Model file for the job. Use its own axes, mm. Give positions to 0.01 mm unless a question says otherwise; leave off trailing zeros. Order: outer loops, then holes, each group sorted by start corner. A loop starts at its lowest first (then second) coordinate and runs counter-clockwise, first axis right, second up. Notation, with made-up numbers: (65.5, 25) - (86.5, 25) arc R23 ccw to (86.5, 43) - close; hole circle Ø9 at (77, 18.25). An arc over 180 degrees is marked (long way). Return JSON: item names as keys, results as strings. Group by question number.
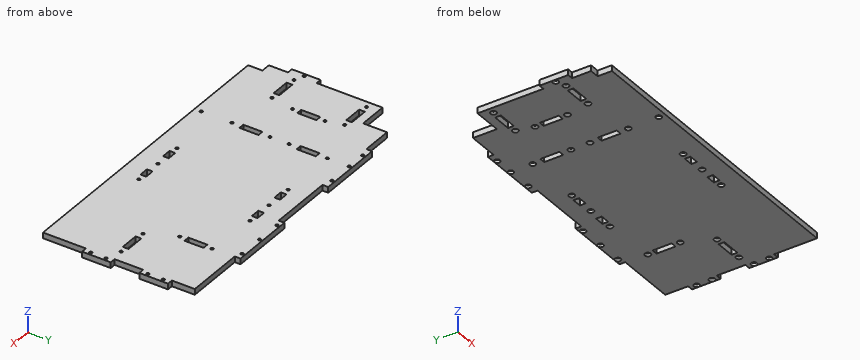
from build123d import *

# Parameters (mm, degrees)
ESQUISSE1_W             = 340
ESQUISSE1_H             = 165
BOSS_EXTRU_1_DEPTH      = 6
ESQUISSE2_W             = 6
ESQUISSE2_H             = 20
ESQUISSE2_W_2           = 68
ESQUISSE2_H_2           = 6
ESQUISSE2_H_3           = 45
ESQUISSE2_H_4           = 35
ESQUISSE2_H_5           = 30
ESQUISSE2_W_3           = 20
ENL_V_MAT_EXTRU_1_DEPTH = 6
ESQUISSE3_W             = 6
ESQUISSE3_H             = 20
ESQUISSE3_W_2           = 20
ESQUISSE3_H_2           = 6
ESQUISSE3_W_3           = 30
ESQUISSE3_H_3           = 25
ENL_V_MAT_EXTRU_2_DEPTH = 10
ESQUISSE5_R             = 1.5
ESQUISSE5_W             = 10
ESQUISSE5_H             = 6
ENL_V_MAT_EXTRU_4_DEPTH = 6
ESQUISSE7_R             = 1.5
ESQUISSE7_R_2           = 1.505
ESQUISSE7_W             = 10
ESQUISSE7_H             = 15
ENL_V_MAT_EXTRU_7_DEPTH = 378.969575495
ESQUISSE8_R             = 2.995
ESQUISSE8_R_2           = 3
ENL_V_MAT_EXTRU_9_DEPTH = 3


with BuildPart() as part:
    # Esquisse1 → Boss.-Extru.1 (new body)
    with BuildSketch(Plane.XY):
        with Locations((-170, 82.5)):
            Rectangle(ESQUISSE1_W, ESQUISSE1_H)
    extrude(amount=BOSS_EXTRU_1_DEPTH)

    # Esquisse2 → Enlèv. mat.-Extru.1 (cut)
    with BuildSketch(Plane.XY.offset(6)):
        Polygon((0, 165), (0, 135), (-6, 135), (-6, 159), (-68, 159), (-68, 165), align=None)
        Polygon((-340, 165), (-272, 165), (-272, 159), (-334, 159), (-334, 65), (-340, 65), align=None)
        with Locations((-67, 119)):
            Rectangle(ESQUISSE2_W, ESQUISSE2_H)
        with Locations((-170, 162)):
            Rectangle(ESQUISSE2_W_2, ESQUISSE2_H_2)
        with Locations((-3, 22.5)):
            Rectangle(ESQUISSE2_W, ESQUISSE2_H_3)
        with Locations((-337, 17.5)):
            Rectangle(ESQUISSE2_W, ESQUISSE2_H_4)
        with Locations((-3, 90)):
            Rectangle(ESQUISSE2_W, ESQUISSE2_H_5)
        with Locations((-36, 73)):
            Rectangle(ESQUISSE2_W_3, ESQUISSE2_H_2)
    extrude(amount=-ENL_V_MAT_EXTRU_1_DEPTH, mode=Mode.SUBTRACT)

    # Esquisse3 → Enlèv. mat.-Extru.2 (cut)
    with BuildSketch(Plane(origin=(0, 0, 0), x_dir=(-1, 0, 0), z_dir=(0, 0, -1))):
        with Locations((241, 119)):
            Rectangle(ESQUISSE3_W, ESQUISSE3_H)
        with Locations((241, 59)):
            Rectangle(ESQUISSE3_W, ESQUISSE3_H)
        with Locations((288.5, 87.5)):
            Rectangle(ESQUISSE3_W, ESQUISSE3_H)
        with Locations((310, 46)):
            Rectangle(ESQUISSE3_W_2, ESQUISSE3_H_2)
        with Locations((310, 122)):
            Rectangle(ESQUISSE3_W_2, ESQUISSE3_H_2)
        with Locations((319, 146.5)):
            Rectangle(ESQUISSE3_W_3, ESQUISSE3_H_3)
    extrude(amount=-ENL_V_MAT_EXTRU_2_DEPTH, mode=Mode.SUBTRACT)

    # Esquisse5 → Enlèv. mat.-Extru.4 (cut)
    with BuildSketch(Plane(origin=(0, 0, 0), x_dir=(-1, 0, 0), z_dir=(0, 0, -1))):
        with Locations((151.5, 138.6)):
            Circle(ESQUISSE5_R)
        with Locations((151.5, 22)):
            Circle(ESQUISSE5_R)
        with Locations((134, 138.6)):
            Rectangle(ESQUISSE5_W, ESQUISSE5_H)
        with Locations((169, 138.6)):
            Rectangle(ESQUISSE5_W, ESQUISSE5_H)
        with Locations((134, 22)):
            Rectangle(ESQUISSE5_W, ESQUISSE5_H)
        with Locations((169, 22)):
            Rectangle(ESQUISSE5_W, ESQUISSE5_H)
    extrude(amount=-ENL_V_MAT_EXTRU_4_DEPTH, mode=Mode.SUBTRACT)

    # Esquisse7 → Enlèv. mat.-Extru.7 (cut, through all)
    with BuildSketch(Plane(origin=(0, 0, 0), x_dir=(-1, 0, 0), z_dir=(0, 0, -1))):
        with Locations((337, 50)):
            Circle(ESQUISSE7_R)
        with Locations((293, 122)):
            Circle(ESQUISSE7_R)
        with Locations((327, 122)):
            Circle(ESQUISSE7_R)
        with Locations((293, 46)):
            Circle(ESQUISSE7_R)
        with Locations((327, 46)):
            Circle(ESQUISSE7_R)
        with Locations((288.5, 70.5)):
            Circle(ESQUISSE7_R)
        with Locations((288.5, 104.5)):
            Circle(ESQUISSE7_R)
        with Locations((241, 39)):
            Circle(ESQUISSE7_R)
        with Locations((241, 79)):
            Circle(ESQUISSE7_R)
        with Locations((241, 99)):
            Circle(ESQUISSE7_R)
        with Locations((241, 139)):
            Circle(ESQUISSE7_R)
        with Locations((241, 7)):
            Circle(ESQUISSE7_R)
        with Locations((241, 162)):
            Circle(ESQUISSE7_R)
        with Locations((262, 162)):
            Circle(ESQUISSE7_R)
        with Locations((214, 162)):
            Circle(ESQUISSE7_R)
        with Locations((75, 162)):
            Circle(ESQUISSE7_R)
        with Locations((102, 162)):
            Circle(ESQUISSE7_R)
        with Locations((129, 162)):
            Circle(ESQUISSE7_R)
        with Locations((67, 102)):
            Circle(ESQUISSE7_R)
        with Locations((67, 136)):
            Circle(ESQUISSE7_R)
        with Locations((53, 73)):
            Circle(ESQUISSE7_R)
        with Locations((19, 73)):
            Circle(ESQUISSE7_R)
        with Locations((3, 52)):
            Circle(ESQUISSE7_R_2)
        with Locations((3, 68)):
            Circle(ESQUISSE7_R)
        with Locations((3, 112)):
            Circle(ESQUISSE7_R)
        with Locations((3, 128)):
            Circle(ESQUISSE7_R)
        with Locations((122, 138.6)):
            Circle(ESQUISSE7_R)
        with Locations((181, 138.6)):
            Circle(ESQUISSE7_R)
        with Locations((181, 22)):
            Circle(ESQUISSE7_R)
        with Locations((122, 22)):
            Circle(ESQUISSE7_R)
        with Locations((329, 7.5)):
            Rectangle(ESQUISSE7_W, ESQUISSE7_H)
    extrude(amount=-ENL_V_MAT_EXTRU_7_DEPTH, mode=Mode.SUBTRACT)

    # Esquisse8 → Enlèv. mat.-Extru.9 (cut)
    with BuildSketch(Plane(origin=(0, 0, 0), x_dir=(-1, 0, 0), z_dir=(0, 0, -1))):
        with Locations((3, 52)):
            Circle(ESQUISSE8_R)
        with Locations((3, 68)):
            Circle(ESQUISSE8_R)
        with Locations((19, 73)):
            Circle(ESQUISSE8_R_2)
        with Locations((3, 112)):
            Circle(ESQUISSE8_R)
        with Locations((3, 128)):
            Circle(ESQUISSE8_R)
        with Locations((53, 73)):
            Circle(ESQUISSE8_R_2)
        with Locations((67, 102)):
            Circle(ESQUISSE8_R_2)
        with Locations((67, 136)):
            Circle(ESQUISSE8_R_2)
        with Locations((75, 162)):
            Circle(ESQUISSE8_R)
        with Locations((102, 162)):
            Circle(ESQUISSE8_R)
        with Locations((129, 162)):
            Circle(ESQUISSE8_R)
        with Locations((122, 138.6)):
            Circle(ESQUISSE8_R_2)
        with Locations((151.5, 138.6)):
            Circle(ESQUISSE8_R_2)
        with Locations((181, 138.6)):
            Circle(ESQUISSE8_R_2)
        with Locations((181, 22)):
            Circle(ESQUISSE8_R_2)
        with Locations((151.5, 22)):
            Circle(ESQUISSE8_R_2)
        with Locations((122, 22)):
            Circle(ESQUISSE8_R_2)
        with Locations((214, 162)):
            Circle(ESQUISSE8_R)
        with Locations((241, 162)):
            Circle(ESQUISSE8_R)
        with Locations((262, 162)):
            Circle(ESQUISSE8_R)
        with Locations((241, 139)):
            Circle(ESQUISSE8_R_2)
        with Locations((241, 99)):
            Circle(ESQUISSE8_R_2)
        with Locations((241, 79)):
            Circle(ESQUISSE8_R_2)
        with Locations((241, 39)):
            Circle(ESQUISSE8_R_2)
        with Locations((241, 7)):
            Circle(ESQUISSE8_R_2)
        with Locations((337, 50)):
            Circle(ESQUISSE8_R)
        with Locations((327, 46)):
            Circle(ESQUISSE8_R_2)
        with Locations((293, 46)):
            Circle(ESQUISSE8_R_2)
        with Locations((288.5, 70.5)):
            Circle(ESQUISSE8_R_2)
        with Locations((288.5, 104.5)):
            Circle(ESQUISSE8_R_2)
        with Locations((293, 122)):
            Circle(ESQUISSE8_R_2)
        with Locations((327, 122)):
            Circle(ESQUISSE8_R_2)
    extrude(amount=-ENL_V_MAT_EXTRU_9_DEPTH, mode=Mode.SUBTRACT)


solid = part.part
(1) Drill centre lines: L1, parallel to Y at x = -181, z = 2.2; L2, parallel to Y at x = -122, z = 1.1; L3, parallel to X at y = 104.5, z = 3.8. Where is each one in solid material? Low to high.
(2) Drop flat-ended pins along their axis: pin 1 Ø2 at (y, z) = (94, 4) entering from +X; pin 2 Ø1.8 at (x, y) = (-241, 7) entering from +Z; pin 3 Ø1.8 at (x, z) = (-330.5, 2) entering from -Y; pin 4 Ø5 at (x, y) = (-241, 162) entering from -Z. Give the stop position or say it passes through.
(3) Slice it at A-A (z = 1.55). State how many separate pieces and enclosed holes the cut face has, and give its area (3 significant figures).
(4) Slice it at B-B (y = 146). Give the cut face in (x, z).
Result set:
{
 "1": {"L1": "y = 0 to 19, 25 to 135.6, 141.6 to 159", "L2": "y = 0 to 19, 25 to 135.6, 141.6 to 165", "L3": "x = -334 to -290, -287 to -6"},
 "2": {"pin 1": "stops at x = -6", "pin 2": "passes through", "pin 3": "stops at y = 15", "pin 4": "stops at z = 3"},
 "3": {"separate pieces": "1", "enclosed holes": "43", "area": "50,600 mm²"},
 "4": {"outline": "(-304, 0) - (-6, 0) - (-6, 6) - (-304, 6) - close"}
}
